Geometry check sheet. Reference: the model listing, model coordinates, mm. Round coordinates to 2 decimals unless told otherwise and drop trailing zeros. Write each loop counter-clockwise with the first axis right and the second up, starting at its lowest first coordinate (ties: lowest second). Pieces come first, ordered by that corner, then holes. Notation, with made-up numbers: (73, 1.5) - (90, 1.5) arc R13 ccw to (90, 10.5) - close; hole circle Ø6 at (72.25, 50.25). An arc over 180 degrees is marked (long way). Return JSON: item names as keys, results as strings. Group by question number.
from build123d import *

# Parameters (mm, degrees)
SKETCH1_R           = 2.6
BOSS_EXTRUDE1_DEPTH = 3.175


with BuildPart() as part:
    # Sketch1 → Boss-Extrude1 (new body)
    with BuildSketch(Plane(origin=(0, 0, 0), x_dir=(1, 0, 0), z_dir=(0, 1, 0))):
        Polygon((47.5, 45), (37.5, 30), (-37.5, 30), (-47.5, 45), (-47.5, 60), (-67.5, 60), (-67.5, 0), (67.5, 0), (67.5, 60), (47.5, 60), align=None)
        with Locations((-37.5, 10)):
            Circle(SKETCH1_R, mode=Mode.SUBTRACT)
        with Locations((-57.5, 10)):
            Circle(SKETCH1_R, mode=Mode.SUBTRACT)
        with Locations((-57.5, 30)):
            Circle(SKETCH1_R, mode=Mode.SUBTRACT)
        with Locations((-57.5, 50)):
            Circle(SKETCH1_R, mode=Mode.SUBTRACT)
        with Locations((57.5, 50)):
            Circle(SKETCH1_R, mode=Mode.SUBTRACT)
        with Locations((57.5, 30)):
            Circle(SKETCH1_R, mode=Mode.SUBTRACT)
        with Locations((57.5, 10)):
            Circle(SKETCH1_R, mode=Mode.SUBTRACT)
        with Locations((37.5, 10)):
            Circle(SKETCH1_R, mode=Mode.SUBTRACT)
    extrude(amount=BOSS_EXTRUDE1_DEPTH)


solid = part.part
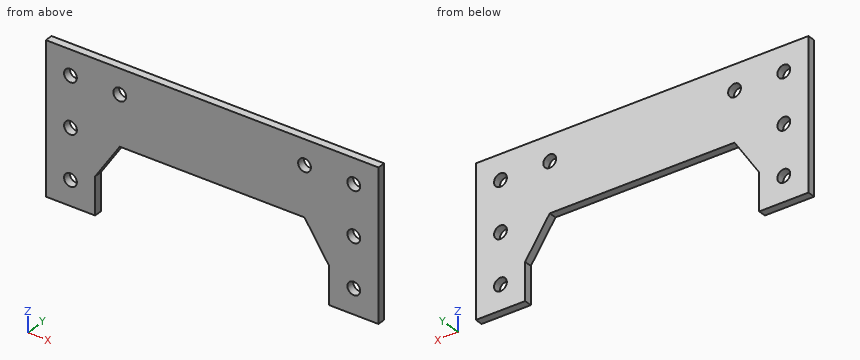
1. Material ranges on line 1 along X through (y, z) = (0.85, -50); line 2 along Z through (x, y) = (57.5, 2.2); line 3 along X through (y, z) = (1.9, -10), recorded low to high.
2. Depth check by flat-ended pin: pin 1 Ø3 at (x, z) = (57.5, -50) entering from +Y; pin 2 Ø1.6 at (x, y) = (18.5, 1) entering from -Z. Enter the tip coordinate at first touch or a pass-through.
3. Section check C-C (y = 1.8). State how many separate pieces and enclosed holes the cut face has, and give its area (3 significant figures).
4. Section check D-D (x = 57.5). Enter the section's corners in (y, z) (3 decimals), and give its area (3 significant figures).
5. Section check B-B (z = -10). Enter the section's corners in (x, y) (3 decimals), and give its area (3 significant figures).
6. Section check A-A (z = -40.5). Enter the section's corners in (x, y) (3 decimals), and give its area (3 significant figures).
Result sheet:
{
 "1": {"line 1": "x = -67.5 to -60.1, -54.9 to -47.5, 47.5 to 54.9, 60.1 to 67.5", "line 2": "z = -60 to -52.6, -47.4 to -32.6, -27.4 to -12.6, -7.4 to 0", "line 3": "x = -67.5 to -60.1, -54.9 to -40.1, -34.9 to 34.9, 40.1 to 54.9, 60.1 to 67.5"},
 "2": {"pin 1": "passes through", "pin 2": "stops at z = -30"},
 "3": {"separate pieces": "1", "enclosed holes": "8", "area": "5,230 mm²"},
 "4": {"outline": "(0, -60) - (3.175, -60) - (3.175, -52.6) - (0, -52.6) - close; (0, -47.4) - (3.175, -47.4) - (3.175, -32.6) - (0, -32.6) - close; (0, -27.4) - (3.175, -27.4) - (3.175, -12.6) - (0, -12.6) - close; (0, -7.4) - (3.175, -7.4) - (3.175, 0) - (0, 0) - close", "area": "141 mm²"},
 "5": {"outline": "(-67.5, 0) - (-60.1, 0) - (-60.1, 3.175) - (-67.5, 3.175) - close; (-54.9, 0) - (-40.1, 0) - (-40.1, 3.175) - (-54.9, 3.175) - close; (-34.9, 0) - (34.9, 0) - (34.9, 3.175) - (-34.9, 3.175) - close; (40.1, 0) - (54.9, 0) - (54.9, 3.175) - (40.1, 3.175) - close; (60.1, 0) - (67.5, 0) - (67.5, 3.175) - (60.1, 3.175) - close", "area": "363 mm²"},
 "6": {"outline": "(-67.5, 0) - (-44.5, 0) - (-44.5, 3.175) - (-67.5, 3.175) - close; (44.5, 0) - (67.5, 0) - (67.5, 3.175) - (44.5, 3.175) - close", "area": "146 mm²"}
}
